from build123d import *

# Parameters (mm, degrees)
F1_DEPTH = 38.1
F2_W     = 19.05
F2_H     = 9.525
F3_DEPTH = 19.05


with BuildPart() as f1:
    # F0 (on Right) → F1 (new body)
    with BuildSketch(Plane.YZ):
        Polygon((152.4, -6.35), (114.3, 19.05), (-114.3, 19.05), (-152.4, -6.35), (-152.4, -19.05), (-101.6, -19.05), (-101.6, -12.7), (101.6, -12.7), (101.6, -19.05), (152.4, -19.05), align=None)
    extrude(amount=F1_DEPTH)

    # F2 (on face) → F3 (cut)
    with BuildSketch(Plane.XY.offset(19.05)):
        with Locations((19.05, 4.7625)):
            Rectangle(F2_W, F2_H)
        with Locations((19.05, -4.7625)):
            Rectangle(F2_W, F2_H)
    extrude(amount=-F3_DEPTH, mode=Mode.SUBTRACT)


with BuildPart() as f4_1:
    # F4: copy of F1
    add(f1.part)


solid = f1.part
Check sheet for the modelled part. Datum: model origin and axes. Units: mm. A direction names the side the tool comes from. Round coordinates to 2 decimals unless told otherwise and drop trailing zeros. Order: outer loops, then holes, each group sorted by start corner. A loop starts at its lowest first (then second) coordinate and runs counter-clockwise, first axis right, second up.
(1) Scan lines: probe 1 along Y at (x, z) = (7.5, -14); probe 2 along Z at (x, y) = (21, -57); probe 3 along Y at (x, z) = (4.5, 11) (3 decimals). Record each from-to range of solid material in increasing order.
(2) Cross-section at D-D, the plane y = 2.5. Enter the section's corners in (x, z) (3 decimals), and give its area (3 significant figures).
(3) Access from +Z, -Z, +X, -X, +Y, -Y to the whole of each face (thin tool, end or side, straight path). Record for faces 5 (the flat face through (19, 9.525, 10)), 6 (the flat face through (19, 101.6, -16)), 7 (the flat face through (38.1, -2, 0)).
(4) Cross-section at A-A, the plane z = -15.5. Enter the section's corners in (x, y).
(5) Draft check along Y on faces 1 (the flat face through (18.78, -133.08, 6.53)), 2 (the flat face through (31, 2, 19.05)), 3 (the flat face through (9.525, 0, 10)), 4 (the flat face through (19, 152.4, -13)). Enter one of: pulls with the +Y half, pulls with the -Y half, needs draft (parallel to the pull), parting line crosses it, or undercut.
(6) Cross-section at C-C, the plane z = 3.5. Enter the section's corners in (x, y) (3 decimals), and give its area (3 significant figures).
(7) Go/stop test with flat-tipped pins: P1, Ø21, axis at x = 18.5, z = 12.5, coming from the +Y side (3 decimals); P2, Ø10, axis at y = -30.5, z = -15, coming from the +X side; P3, Ø10, axis at x = 28, z = 6.5, coming from the -Y side (3 decimals); P4, Ø11.5, axis at x = 27.5, y = 35.5, coming from the -Z side. Record where each tip stops, or that it passes through.
(8) Cross-section at B-B, the plane x = 22. Enter the section's corners in (y, z) (3 decimals), and give its area (3 significant figures).
Check sheet entries:
1. probe 1: y = -152.4 to -101.6, 101.6 to 152.4
1. probe 2: z = -12.7 to 19.05
1. probe 3: y = -126.375 to 126.375
2. outline: (0, -12.7) - (38.1, -12.7) - (38.1, 19.05) - (28.575, 19.05) - (28.575, 0) - (9.525, 0) - (9.525, 19.05) - (0, 19.05) - close
2. area: 847 mm2
3. face 5: +Z
3. face 6: -Z, +X, -X
3. face 7: +Z, -Z, +X, +Y, -Y
4. outline: (0, -152.4) - (38.1, -152.4) - (38.1, -101.6) - (0, -101.6) - close; (0, 101.6) - (38.1, 101.6) - (38.1, 152.4) - (0, 152.4) - close
5. face 1: pulls with the -Y half
5. face 2: needs draft
5. face 3: undercut
5. face 4: pulls with the +Y half
6. outline: (0, -137.625) - (38.1, -137.625) - (38.1, 137.625) - (0, 137.625) - close; hole (9.525, -9.525) - (28.575, -9.525) - (28.575, 9.525) - (9.525, 9.525) - close
6. area: 10,100 mm2
7. P1: stops at y = 139.875
7. P2: stops at x = 38.1
7. P3: stops at y = -140.625
7. P4: stops at z = -12.7
8. outline: (-152.4, -19.05) - (-101.6, -19.05) - (-101.6, -12.7) - (101.6, -12.7) - (101.6, -19.05) - (152.4, -19.05) - (152.4, -6.35) - (114.3, 19.05) - (9.525, 19.05) - (9.525, 0) - (-9.525, 0) - (-9.525, 19.05) - (-114.3, 19.05) - (-152.4, -6.35) - close
8. area: 8,990 mm2
